Job drawing, mm, ordinate dimensions from the low corner. One solid piece. A direction names the side the tool comes from. Coordinates: 2 decimals unless noted, no trailing zeros. Write each loop counter-clockwise with the first axis right and the second up, starting at its lowest first coordinate (ties: lowest second). Pieces come first, ordered by that corner, then holes. Notation, with made-up numbers: (-8, -32) - (36, -32) arc R17 ccw to (36, -13) - close; hole circle Ø8 at (-35.5, -40). An arc over 180 degrees is marked (long way). Put each result on its own line as item: value. Start each with the question number.
1. Pull direction X, two halves, no side cores. Call the marked faces 1, 2 and 3: released by +X, released by -X, zero draft, split by the parting line, or undercut.
2. Saw through at B-B, the plane y = 13.75. Write the cut outline in (x, z).
3. Saw through at A-A, the plane z = 12.5. Write the cut outline in (x, y).
4. Saw through at C-C, the plane x = 12.5. Write the cut outline in (y, z).
5. Drill centre lines: L1, parallel to Y at x = 19, z = 2; L2, parallel to Z at x = 37.5, y = 10.25; L3, parallel to X at y = 11.25, z = 11.75. Where is each one in solid material? Low to high. Write a range as from..to.
6. Which spindle directions (+Z, -Z, +X, -X, +Y, -Y) get a long thin tool onto all of the face, cutting with end or side? Do the marked faces 4 and 5. Say none if no direction does.
7. Saw through at D-D, the plane z = 16.75. Write the cut outline in (x, y), plus the area to 3 significant figures.
8. Drop flat-ended pins along their axis: P1, Ø3, axis at y = 12.5, z = 11, coming from the +X side; P2, Ø3, axis at y = 3, z = 20, coming from the -X side; P3, Ø4, axis at y = 13, z = 8.5, coming from the +X side. Give the stop position or say it passes through.
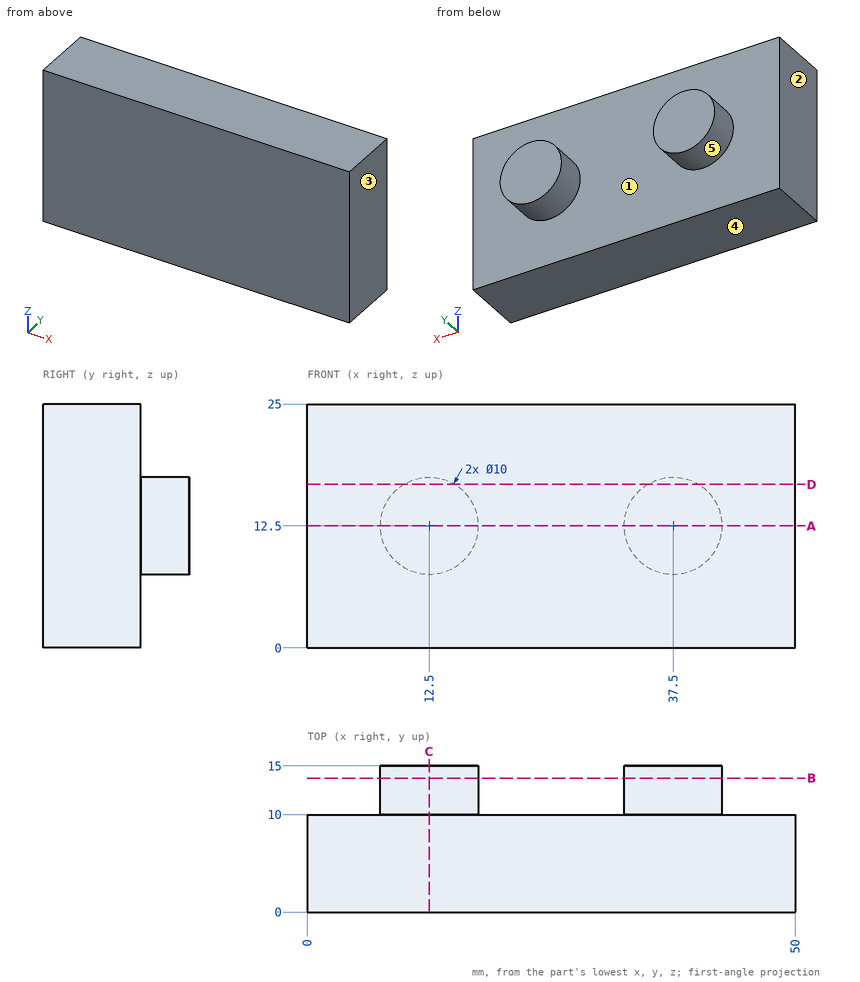
Final values:
1. face 1: undercut
1. face 2: released by -X
1. face 3: released by +X
2. outline: circle Ø10 at (12.5, 12.5); circle Ø10 at (37.5, 12.5)
3. outline: (0, 0) - (50, 0) - (50, 10) - (42.5, 10) - (42.5, 15) - (32.5, 15) - (32.5, 10) - (17.5, 10) - (17.5, 15) - (7.5, 15) - (7.5, 10) - (0, 10) - close
4. outline: (0, 0) - (10, 0) - (10, 7.5) - (15, 7.5) - (15, 17.5) - (10, 17.5) - (10, 25) - (0, 25) - close
5. L1: y = 0..10
5. L2: z = 7.5..17.5
5. L3: x = 7.56..17.44, 32.56..42.44
6. face 4: -Z, +X, -X, +Y, -Y
6. face 5: +Y
7. outline: (0, 0) - (50, 0) - (50, 10) - (40.13, 10) - (40.13, 15) - (34.87, 15) - (34.87, 10) - (15.13, 10) - (15.13, 15) - (9.87, 15) - (9.87, 10) - (0, 10) - close
7. area: 553 mm²
8. P1: stops at x = 42.5
8. P2: stops at x = 0
8. P3: stops at x = 42.08
